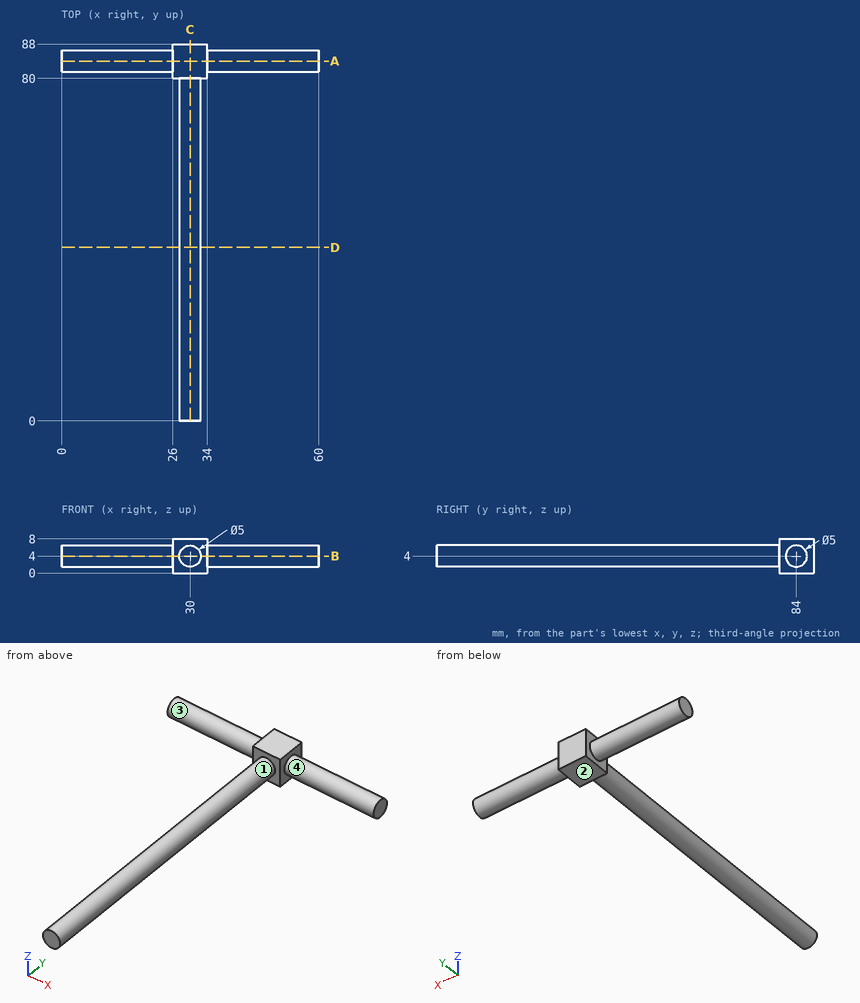
Check sheet for the drawn part. Datum: minimum x, y, z corner. Units: mm. A direction names the side the tool comes from. Coordinates: 2 decimals unless noted, no trailing zeros. Order: outer loops, then holes, each group sorted by start corner. A loop starts at its lowest first (then second) coordinate and runs counter-clockwise, first axis right, second up. Notation, with made-up numbers: M 17,-24 L 42,-24 A24 ccw 42,14 Z; hole C -23,-12 d10. An arc over 180 degrees is marked long. One line per question, with ' | ' between items. Start each with the question number.
Item 1: Cross-section at A-A on y = 84. Enter the section's corners in (x, z), then the cut area to 3 significant figures.
Item 2: Set-up check for the marked faces 1, 2, 3 and 4: record each of +Z, -Z, +X, -X, +Y, -Y from which the full face is reachable in a straight line by a thin tool's end or side.
Item 3: Material ranges on L1, parallel to X at y = 37, z = 4; L2, parallel to Y at x = 28.5, z = 7.5; L3, parallel to Z at x = 32, y = 37, recorded low to high. Write a range as [from, to].
Item 4: Cross-section at D-D on y = 40.5. Enter the section's corners in (x, z), then the cut area to 3 significant figures.
Item 5: Cross-section at C-C on x = 30. Enter the section's corners in (y, z).
Item 6: Gauge pin test, flat ends, axial feed: pin 1 (1 mm diameter, centred on x = 13.5, z = 5.5, fed in from -Y); pin 2 (2 mm diameter, centred on y = 21.5, z = 6.5, fed in from -X); pin 3 (4 mm diameter, centred on y = 45.5, z = 2, fed in from -X). Record the tip position at first contact, or that the pin passes through.
Item 7: Cross-section at B-B on z = 4. Enter the section's corners in (x, y), then the cut area to 3 significant figures.
Findings:
1) outline: M 0,1.5 L 26,1.5 L 26,0 L 34,0 L 34,1.5 L 60,1.5 L 60,6.5 L 34,6.5 L 34,8 L 26,8 L 26,6.5 L 0,6.5 Z | area: 324 mm²
2) face 1: -Y | face 2: -Z, +X, -X, +Y, -Y | face 3: -X | face 4: +X
3) L1: x = [27.5, 32.5] | L2: y = [80, 88] | L3: z = [2.5, 5.5]
4) outline: C 30,4 d5 | area: 19.6 mm²
5) outline: M 0,1.5 L 80,1.5 L 80,0 L 88,0 L 88,8 L 80,8 L 80,6.5 L 0,6.5 Z
6) pin 1: stops at y = 81.71 | pin 2: stops at x = 28 | pin 3: stops at x = 27.5
7) outline: M 0,81.5 L 26,81.5 L 26,80 L 27.5,80 L 27.5,0 L 32.5,0 L 32.5,80 L 34,80 L 34,81.5 L 60,81.5 L 60,86.5 L 34,86.5 L 34,88 L 26,88 L 26,86.5 L 0,86.5 Z | area: 724 mm²
